Geometry check sheet. Reference: the model listing, model coordinates, mm. A direction names the side the tool comes from. Round coordinates to 2 decimals unless told otherwise and drop trailing zeros. Write each loop counter-clockwise with the first axis right and the second up, starting at its lowest first coordinate (ties: lowest second). Pieces come first, ordered by that corner, then holes. Notation, with made-up numbers: M 88,-14 L 130,-14 A30 cw 130,19 Z; hole C 77.25,0 d6. An arc over 180 degrees is marked long. Answer as CSV lines item,"result". Start each with the question number.
```python
from build123d import *

# Parameters (mm, degrees)
BOSS_EXTRUDE1_DEPTH     = 392
CUT_EXTRUDE1_DEPTH      = 396.116955248
CUT_EXTRUDE1_DEPTH_BACK = 396.116955248
SKETCH2_W               = 4
SKETCH2_H               = 36
CUT_EXTRUDE2_DEPTH      = 400.775227771
CUT_EXTRUDE2_DEPTH_BACK = 400.775227771
SKETCH3_R               = 7.5


with BuildPart() as part:
    # Sketch1 → Boss-Extrude1 (new body)
    with BuildSketch(Plane(origin=(0, 0, 0), x_dir=(1, 0, 0), z_dir=(0, 1, 0))):
        with BuildLine():
            Line((-27.499872145, 29.213153277), (-67.499872145, 29.213153277))
            Line((-67.499872145, 29.213153277), (-67.499872145, -10.786846723))
            Line((-67.499872145, -10.786846723), (-66.499872145, -10.786846723))
            ThreePointArc((-66.499872145, -10.786846723), (-64.378551801, -9.908167067), (-63.499872145, -7.786846723))
            Line((-63.499872145, -7.786846723), (-63.499872145, 22.213153277))
            ThreePointArc((-63.499872145, 22.213153277), (-62.621192489, 24.334473621), (-60.499872145, 25.213153277))
            Line((-60.499872145, 25.213153277), (-30.499872145, 25.213153277))
            ThreePointArc((-30.499872145, 25.213153277), (-28.378551801, 26.091832933), (-27.499872145, 28.213153277))
            Line((-27.499872145, 28.213153277), (-27.499872145, 29.213153277))
        make_face()
    extrude(amount=BOSS_EXTRUDE1_DEPTH)

    # Sketch2 → Cut-Extrude1 (cut, two sides: drawn at the far end of the back side and taken through both)
    with BuildSketch(Plane.ZY.offset(67.499872145).offset(-CUT_EXTRUDE1_DEPTH_BACK)):
        with Locations((-27.213153277, 374)):
            Rectangle(SKETCH2_W, SKETCH2_H)
        with Locations((-27.213153277, 18)):
            Rectangle(SKETCH2_W, SKETCH2_H)
    extrude(amount=CUT_EXTRUDE1_DEPTH + CUT_EXTRUDE1_DEPTH_BACK, mode=Mode.SUBTRACT)

    # Sketch3 → Cut-Extrude2 (cut, two sides: drawn at the far end of the back side and taken through both)
    with BuildSketch(Plane(origin=(0, 0, -29.213153277), x_dir=(-1, 0, 0), z_dir=(0, 0, -1)).offset(-CUT_EXTRUDE2_DEPTH_BACK)):
        with Locations((49.390570274, 323)):
            Circle(SKETCH3_R)
        with Locations((49.390570274, 69)):
            Circle(SKETCH3_R)
    extrude(amount=CUT_EXTRUDE2_DEPTH + CUT_EXTRUDE2_DEPTH_BACK, mode=Mode.SUBTRACT)


solid = part.part
```
1) Go/stop test with flat-tipped pins: pin 1 (8 mm diameter, centred on y = 127, z = -4, fed in from +X); pin 2 (24 mm diameter, centred on x = -52.5, y = 121, fed in from +Z); pin 3 (4.5 mm diameter, centred on x = -45.5, z = -27, fed in from -Y). Record where each tip stops, or that it passes through.
2) Mould release check, pull along X, two halves, no side actions. Record for faces 1 (the cylindrical face through (-47.76, 315.68, -27.19)), 2 (the flat face through (-64, 18, -25.213)), 3 (the flat face through (-63.5, 193, -7)): released by +X, released by -X, zero draft, split by the parting line, or undercut.
3) Scan lines: line 1 (X direction, y = 336, z = 7.5); line 2 (Z direction, x = -55, y = 234); line 3 (X direction, y = 69, z = -27). Record each from-to range of solid material in increasing order. Write a range as from..to.
4) Section check C-C, the plane x = -35.5. Record the cut outline in (y, z).
5) Section check D-D, the plane z = -7. Record the cut outline in (x, y).
6) Section check B-B, the plane y = 45. Record the cut outline in (x, z).
7) Section check A-A, the plane y = 323. Record the cut outline in (x, z).
8) Access from +Z, -Z, +X, -X, +Y, -Y to the whole of each face (thin tool, end or side, straight path). Record for faces 4 (the flat face through (-64, 374, -25.213)), 5 (the flat face through (-47, 194, -29.213)), 6 (the flat face through (-46, 194, -25.213)).
Results:
1,pin 1,"stops at x = -63.5"
1,pin 2,"stops at z = 10.02"
1,pin 3,"stops at y = 36"
2,face 1,"undercut"
2,face 2,"zero draft"
2,face 3,"released by +X"
3,line 1,"x = -67.5..-63.5"
3,line 2,"z = -29.21..-25.21"
3,line 3,"x = -67.5..-56.89, -41.89..-27.76"
4,outline,"M 36,-29.21 L 356,-29.21 L 356,-25.21 L 36,-25.21 Z"
5,outline,"M -67.5,0 L -63.5,0 L -63.5,392 L -67.5,392 Z"
6,outline,"M -67.5,-29.21 L -27.5,-29.21 L -27.5,-28.21 A3 ccw -30.5,-25.21 L -60.5,-25.21 A3 cw -63.5,-22.21 L -63.5,7.79 A3 ccw -66.5,10.79 L -67.5,10.79 Z"
7,outline,"M -67.5,-29.21 L -56.89,-29.21 L -56.89,-25.21 L -60.5,-25.21 A3 cw -63.5,-22.21 L -63.5,7.79 A3 ccw -66.5,10.79 L -67.5,10.79 Z; M -41.89,-29.21 L -27.5,-29.21 L -27.5,-28.21 A3 ccw -30.5,-25.21 L -41.89,-25.21 Z"
8,face 4,"-Z, +X, -X, +Y"
8,face 5,"-Z, +X, -X, +Y, -Y"
8,face 6,"+Z, +X, +Y, -Y"
